from build123d import *

# Parameters (mm, degrees)
SKETCH2_R                            = 4.85
CUT_EXTRUDE1_DEPTH                   = 9
SKETCH3_R                            = 3.5
BOSS_EXTRUDE1_DEPTH                  = 2
BOSS_EXTRUDE1_DIRECTION_2_REACH      = 78.487
BOSS_EXTRUDE1_DIRECTION_2_END_RADIUS = 16.5


with BuildPart() as part:
    # Sketch1 → Revolve1 (revolve)
    with BuildSketch(Plane(origin=(0, 0, 0), x_dir=(1, 0, 0), z_dir=(0, 1, 0)), mode=Mode.PRIVATE) as revolve1_sk:
        Polygon((0, 10), (0, 6), (2, 4), (11, 4), (11, 0), (67, 0), (67, 4), (64, 4), (64, 16.5), (9, 16.5), (9, 11), (1, 11), align=None)
    revolve(revolve1_sk.sketch.rotate(Axis((0, 0, 0), (1, 0, 0)), 180), axis=Axis((0, 0, 0), (1, 0, 0)))

    # Sketch2 → Cut-Extrude1 (cut)
    with BuildSketch(Plane.XY.offset(16.5)):
        with Locations((25, 0)):
            Circle(SKETCH2_R)
    extrude(amount=-CUT_EXTRUDE1_DEPTH, mode=Mode.SUBTRACT)


with BuildPart() as boss_extrude1_tool:
    # Sketch3 → Boss-Extrude1 (new body)
    with BuildSketch(Plane.XY.offset(16.5)):
        with Locations((39, 0)):
            Circle(SKETCH3_R)
    extrude(amount=BOSS_EXTRUDE1_DEPTH)


with BuildPart() as part_1:
    add(part.part)


with BuildPart() as part_2:
    # Boss-Extrude1: joined with boss_extrude1_tool
    add(part_1.part.fuse(boss_extrude1_tool.part, tol=0.00001))

    # Boss-Extrude1 direction 2: up to this cylinder (the profile starts outside it)
    boss_extrude1_direction_2_end = Plane(origin=(39, 0, 0), z_dir=(-1, 0, 0)) * Cylinder(BOSS_EXTRUDE1_DIRECTION_2_END_RADIUS, 190.974, mode=Mode.PRIVATE)
    # Sketch3 → Boss-Extrude1 direction 2 (add, up to the surface)
    with BuildSketch(Plane.XY.offset(16.5), mode=Mode.PRIVATE) as boss_extrude1_direction_2_sk1:
        with Locations((39, 0)):
            Circle(SKETCH3_R)
    boss_extrude1_direction_2_tool1 = extrude(boss_extrude1_direction_2_sk1.sketch, amount=-BOSS_EXTRUDE1_DIRECTION_2_REACH, mode=Mode.PRIVATE) - boss_extrude1_direction_2_end
    add(boss_extrude1_direction_2_tool1.solids().sort_by_distance((39, 0, 16.5))[0])
    add(boss_extrude1_direction_2_tool1.solids().sort_by_distance((39, 0, 16.5))[1])


solid = part_2.part
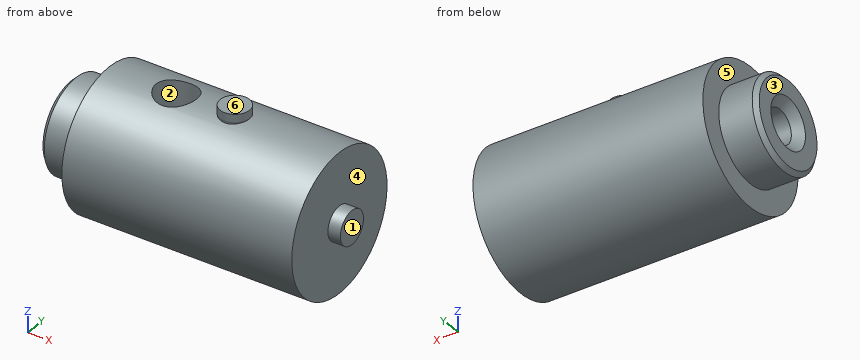
Here's how the part is built. I have some questions about the finished solid (model axes, mm). Face numbers are marked on the shaded views. A direction names the side the tool comes from. Give positions to 0.01 mm unless a question says otherwise; leave off trailing zeros. Write each loop counter-clockwise with the first axis right and the second up, starting at its lowest first coordinate (ties: lowest second). Pieces come first, ordered by that corner, then holes. Notation, with made-up numbers: (66.25, 73.5) -> (84.25, 73.5) arc R18 cw to (84.25, 90.5) -> close; hole circle Ø2 at (55, 49). An arc over 180 degrees is marked (long way). Use one line per item in the form item = value. Start each with the question number.
1. On a 3-axis mill with a long thin cutter (end or side, diameter ignored), from which of +Z, -Z, +X, -X, +Y, -Y can I reach the whole of each face in a straight line? I mean the marked faces 4, 5 and 6. Say none if no direction works.
2. Thinking about a two-plate mould opening in X: for the marked faces 1, 2 and 3, which applies, +X half, -X half, draft (parallel to the pull), parting line (faces both ways), or undercut?
3. Imagine slicing it at D-D on x = 57.5. List the corners of the cut face in (y, z) for me.
4. If I drill on L1, parallel to Y at x = 9.25, z = 0; L2, parallel to Y at x = 6.5, z = 0; L3, parallel to X at y = 8, z = 9, over which ranges is the centre line in solid material (lowest first)?
5. Will these pins go through, and if not, where does the flat tip stop? pin 1 Ø6 at (x, y) = (24, 7.5) entering from +Z; pin 2 Ø8 at (x, z) = (35.5, 13) entering from -Y; pin 3 Ø8 at (x, z) = (60, 14.5) entering from -Y.
6. Imagine slicing it at B-B on z = 0. List the corners of the cut face in (x, y) for me.
7. Imagine slicing it at C-C on y = 12. List the corners of the cut face in (x, z) for me, plus the area to 3 significant figures.
8. Imagine slicing it at A-A on x = 6.5. List the corners of the cut face in (y, z) for me.
Entries:
q1.face_4 = +X
q1.face_5 = -X
q1.face_6 = +Z, +X, -X, +Y, -Y
q2.face_1 = +X half
q2.face_2 = undercut
q2.face_3 = -X half
q3.outline = circle Ø33 at (0, 0)
q4.L1 = -16.5 to -4, 4 to 16.5
q4.L2 = -11 to -4, 4 to 11
q4.L3 = 9 to 64
q5.pin_1 = 15.86
q5.pin_2 = -13.83
q5.pin_3 = -12.73
q6.outline = (0, -10) -> (1, -11) -> (9, -11) -> (9, -16.5) -> (64, -16.5) -> (64, -4) -> (67, -4) -> (67, 4) -> (64, 4) -> (64, 16.5) -> (9, 16.5) -> (9, 11) -> (1, 11) -> (0, 10) -> (0, 6) -> (2, 4) -> (11, 4) -> (11, -4) -> (2, -4) -> (0, -6) -> close
q7.outline = (9, -11.32) -> (64, -11.32) -> (64, 11.32) -> (9, 11.32) -> close
q7.area = 1,250 mm²
q8.outline = circle Ø22 at (0, 0); hole circle Ø8 at (0, 0)
